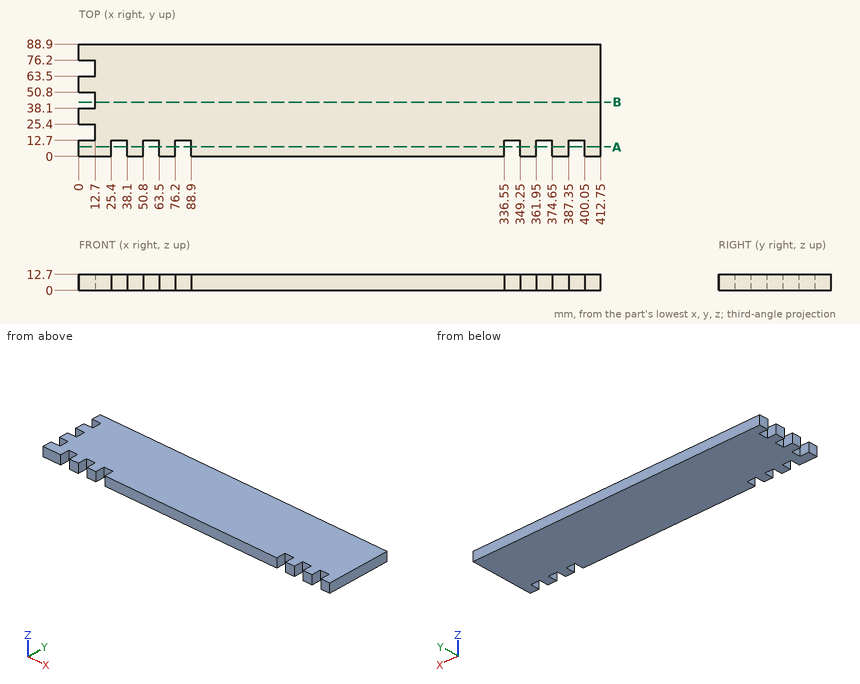
Here's the drawing with two shaded views (mm, measured from the low corner). I have some questions. Give positions to 0.01 mm unless a question says otherwise; leave off trailing zeros. Loops run counter-clockwise (first coordinate to the right, second up) from the corner with the lowest first, then second, coordinate; pieces in that order, holes last. Notation, with made-up numbers: M 46.5,36 L 55.5,36 A17 ccw 55.5,58 Z; hole C 11,49 d3. An arc over 180 degrees is marked long. Answer in a Markdown table with one row per item.
1. Suppose I cut it at A-A on y = 7.5. Write out the boundary of the cut face in (x, z), plus the area to 3 significant figures.
Taken from the geometry:
| item | result |
|---|---|
| outline | M 0,0 L 25.4,0 L 25.4,12.7 L 0,12.7 Z; M 38.1,0 L 50.8,0 L 50.8,12.7 L 38.1,12.7 Z; M 63.5,0 L 76.2,0 L 76.2,12.7 L 63.5,12.7 Z; M 88.9,0 L 336.55,0 L 336.55,12.7 L 88.9,12.7 Z; M 349.25,0 L 361.95,0 L 361.95,12.7 L 349.25,12.7 Z; M 374.65,0 L 387.35,0 L 387.35,12.7 L 374.65,12.7 Z; M 400.05,0 L 412.75,0 L 412.75,12.7 L 400.05,12.7 Z |
| area | 4,270 mm² |
2. If I drill on line 1 along X through (y, z) = (75.5, 9); line 2 along Y through (x, z) = (347, 11.25), over which ranges is the centre line in solid material (lowest first)?
Taken from the geometry:
| item | result |
|---|---|
| line 1 | x = 12.7 to 412.75 |
| line 2 | y = 12.7 to 88.9 |
3. Suppose I cut it at B-B on y = 43. Write out the boundary of the cut face in (x, z), plus the area to 3 significant figures.
Taken from the geometry:
| item | result |
|---|---|
| outline | M 12.7,0 L 412.75,0 L 412.75,12.7 L 12.7,12.7 Z |
| area | 5,080 mm² |
4. For pin 1 Ø6.5 at (x, z) = (342.5, 8.5) entering from -Y; pin 2 Ø6.5 at (y, z) = (16, 6.5) entering from -X, each with a flat end and sliding along its axis, tell me the tip position at first contact or that it passes through.
Taken from the geometry:
| item | result |
|---|---|
| pin 1 | stops at y = 12.7 |
| pin 2 | stops at x = 12.7 |
